Geometry check sheet. Reference: the model listing, model coordinates, mm. A direction names the side the tool comes from. Coordinates: 2 decimals unless noted, no trailing zeros. Write each loop counter-clockwise with the first axis right and the second up, starting at its lowest first coordinate (ties: lowest second). Pieces come first, ordered by that corner, then holes. Notation, with made-up numbers: M -11,-7.5 L 32,-7.5 A17 cw 32,11.5 Z; hole C 58,-37.5 d11. An arc over 180 degrees is marked long. Write each question's results on one line, items separated by ' | '.
```python
from build123d import *

# Parameters (mm, degrees)
F0_W     = 65
F0_H     = 11
F1_DEPTH = 2160
F2_W     = 615
F2_H     = 920
F3_DEPTH = 50
F2_W_2   = 470
F2_H_2   = 59.696319
F4_DEPTH = 850
F5_W     = 695
F5_H     = 190
F6_DEPTH = 60
F7_DEPTH = 400


with BuildPart() as f1:
    # F0 (on Top) → F1 (new body)
    with BuildSketch(Plane.XY):
        Polygon((-570.886376, 90.884483), (-570.886376, 899.884483), (974.113624, 899.884483), (974.113624, 79.884483), (299.113624, 79.884483), (234.113624, 79.884483), (234.113624, 19.884483), (1034.113624, 19.884483), (1034.113624, 959.884483), (-630.886376, 959.884483), (-630.886376, 19.884483), (-570.886376, 19.884483), (-570.886376, 79.884483), align=None)
        Polygon((-460.886376, 90.884483), (-570.886376, 90.884483), (-570.886376, 79.884483), (-570.886376, 19.884483), (-460.886376, 19.884483), align=None)
        with Locations((266.613624, 85.384483)):
            Rectangle(F0_W, F0_H)
    extrude(amount=F1_DEPTH)

    # F2 (on face) → F3 (cut)
    with BuildSketch(Plane.XZ.offset(-899.884483)):
        with Locations((-33.386376, 1600)):
            Rectangle(F2_W, F2_H)
    extrude(amount=-F3_DEPTH, mode=Mode.SUBTRACT)

    # F2 (on face) → F4 (join)
    with BuildSketch(Plane.XZ.offset(-899.884483)):
        with Locations((739.113624, 739.84816)):
            Rectangle(F2_W_2, F2_H_2)
    extrude(amount=F4_DEPTH)

    # F5 (on face) → F6 (join)
    with BuildSketch(Plane.XZ.offset(-19.884483)):
        with Locations((-113.386376, 2065)):
            Rectangle(F5_W, F5_H)
    extrude(amount=-F6_DEPTH)

    # F2 (on face) → F7 (join)
    with BuildSketch(Plane.XZ.offset(-899.884483)):
        Polygon((974.113624, 797.217071), (-570.886376, 797.217071), (-570.886376, 769.696319), (504.113624, 769.696319), (974.113624, 769.696319), align=None)
    extrude(amount=F7_DEPTH)


solid = f1.part
```
Q1. Sectioned sample at C-C on y = 298. Record the cut outline in (x, z).
Geometry check:
outline: M -630.89,0 L -570.89,0 L -570.89,2160 L -630.89,2160 Z; M 504.11,710 L 974.11,710 L 974.11,0 L 1034.11,0 L 1034.11,2160 L 974.11,2160 L 974.11,769.7 L 504.11,769.7 Z
Q2. Sectioned sample at B-B on z = 354.5. Record the cut outline in (x, y).
Geometry check:
outline: M -630.89,19.88 L -460.89,19.88 L -460.89,90.88 L -570.89,90.88 L -570.89,899.88 L 974.11,899.88 L 974.11,79.88 L 299.11,79.88 L 299.11,90.88 L 234.11,90.88 L 234.11,19.88 L 1034.11,19.88 L 1034.11,959.88 L -630.89,959.88 Z
Q3. Sectioned sample at A-A on x = -530. Record the cut outline in (y, z).
Geometry check:
outline: M 19.88,0 L 90.88,0 L 90.88,2160 L 19.88,2160 Z; M 499.88,769.7 L 899.88,769.7 L 899.88,0 L 959.88,0 L 959.88,2160 L 899.88,2160 L 899.88,797.22 L 499.88,797.22 Z
Q4. Scan lines: probe 1 along X at (y, z) = (89.5, 1190.5); probe 2 along Y at (x, z) = (533.5, 1984); probe 3 along X at (y, z) = (78, 1271.5). Record each from-to range of solid material in increasing order.
Geometry check:
probe 1: x = -630.89 to -460.89, 234.11 to 299.11, 974.11 to 1034.11 | probe 2: y = 19.88 to 79.88, 899.88 to 959.88 | probe 3: x = -630.89 to -460.89, 234.11 to 1034.11
Q5. Sectioned sample at D-D on z = 2008.5. Record the cut outline in (x, y), and give its area (3 significant figures).
Geometry check:
outline: M -630.89,19.88 L 1034.11,19.88 L 1034.11,959.88 L -630.89,959.88 Z; hole M -570.89,90.88 L -460.89,90.88 L -460.89,79.88 L 234.11,79.88 L 234.11,90.88 L 299.11,90.88 L 299.11,79.88 L 974.11,79.88 L 974.11,899.88 L 274.11,899.88 L 274.11,949.88 L -340.89,949.88 L -340.89,899.88 L -570.89,899.88 Z | area: 269,000 mm2
Q6. Depth check by flat-ended pin: P1, Ø8, axis at x = 199.5, y = 737.5, coming from the -Z side; P2, Ø1.5, axis at x = -197.5, z = 431, coming from the -Y side; P3, Ø1.5, axis at x = 159.5, y = 558, coming from the +Z side. Enter the tip coordinate at first touch or a pass-through.
Geometry check:
P1: stops at z = 769.7 | P2: stops at y = 899.88 | P3: stops at z = 797.22
Q7. Access from +Z, -Z, +X, -X, +Y, -Y to the whole of each face (thin tool, end or side, straight path). Record for faces 1 (the flat face through (736, 293, 769.696)), 2 (the flat face through (974.114, 496, 350)), 3 (the flat face through (-38, 925, 2060)).
Geometry check:
face 1: +Z | face 2: -Z | face 3: none
Q8. Mould release check, pull along X, two halves, no side actions. Record for faces 4 (the flat face through (213, 959.884, 1065)), 5 (the flat face through (736, 496, 710)), 6 (the flat face through (1034.114, 483, 1065)): pulls with the +X half, pulls with the -X half, needs draft (parallel to the pull), parting line crosses it, or undercut.
Geometry check:
face 4: needs draft | face 5: undercut | face 6: pulls with the +X half
